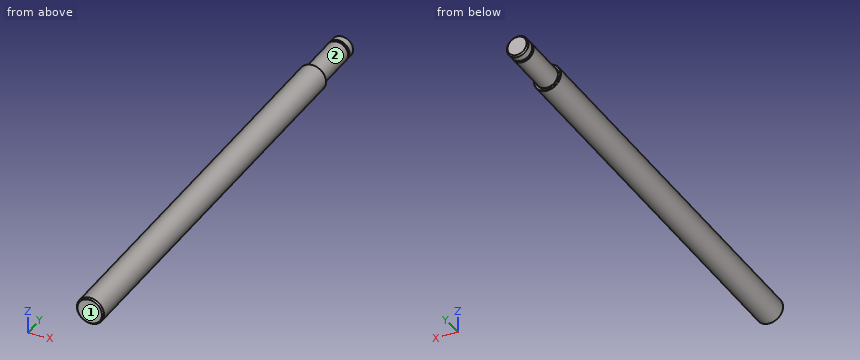
from build123d import *

# Parameters (mm, degrees)
RESSALTO_EXTRUS_O1_DEPTH      = 94
RESSALTO_EXTRUS_O1_DEPTH_BACK = 82
ESBO_O1_R                     = 5
ESBO_O2_R                     = 14
ESBO_O2_R_2                   = 4
CORTE_EXTRUS_O1_DEPTH         = 21
CHANFRO1_SIZE                 = 0.5
FILETE1_R                     = 0.25
CHANFRO2_SIZE                 = 0.5
CORTE_EXTRUS_O2_START         = -3
ESBO_O3_R                     = 13.5
ESBO_O3_R_2                   = 3.5
CORTE_EXTRUS_O2_DEPTH         = 1


with BuildPart() as part:
    # Esboço1 → Ressalto-extrusão1 (new, two sides: drawn at the far end of the back side and taken through both)
    with BuildSketch(Plane(origin=(0, 0, 0), x_dir=(1, 0, 0), z_dir=(0, 1, 0)).offset(-RESSALTO_EXTRUS_O1_DEPTH_BACK)):
        with Locations(Location((0, 0, 0), (0, 0, 270))):
            Circle(ESBO_O1_R)
    extrude(amount=RESSALTO_EXTRUS_O1_DEPTH + RESSALTO_EXTRUS_O1_DEPTH_BACK)

    # Esboço2 → Corte-extrusão1 (cut)
    with BuildSketch(Plane(origin=(0, 94, 0), x_dir=(1, 0, 0), z_dir=(0, 1, 0))):
        Circle(ESBO_O2_R)
        with Locations(Location((0, 0, 0), (0, 0, 270))):
            Circle(ESBO_O2_R_2, mode=Mode.SUBTRACT)
    extrude(amount=-CORTE_EXTRUS_O1_DEPTH, mode=Mode.SUBTRACT)

    # Chanfro1
    chanfro1_edges = [part.edges().sort_by_distance(p)[0] for p in [
        (0, 94, -4),
    ]]
    chamfer(chanfro1_edges, length=CHANFRO1_SIZE)

    # Filete1
    filete1_edges = [part.edges().sort_by_distance(p)[0] for p in [
        (0, 73, -5),
        (0, 73, -4),
    ]]
    fillet(filete1_edges, radius=FILETE1_R)

    # Chanfro2
    chanfro2_edges = [part.edges().sort_by_distance(p)[0] for p in [
        (0, -82, -5),
    ]]
    chamfer(chanfro2_edges, length=CHANFRO2_SIZE)

    # Esboço3 → Corte-extrusão2 (cut)
    with BuildSketch(Plane(origin=(0, 94, 0), x_dir=(1, 0, 0), z_dir=(0, 1, 0)).offset(CORTE_EXTRUS_O2_START)):
        Circle(ESBO_O3_R)
        with Locations(Location((0, 0, 0), (0, 0, 270))):
            Circle(ESBO_O3_R_2, mode=Mode.SUBTRACT)
    extrude(amount=-CORTE_EXTRUS_O2_DEPTH, mode=Mode.SUBTRACT)


solid = part.part
For this review, take the finished solid that the model builds, in its own axes (mm). Face numbers are marked on the shaded views. A direction names the side the tool comes from. Coordinates: 2 decimals unless noted, no trailing zeros. Loops run counter-clockwise (first coordinate to the right, second up) from the corner with the lowest first, then second, coordinate; pieces in that order, holes last. Notation, with made-up numbers: (-18, 53) - (10, 53) arc R28 cw to (10, 83) - close; hole circle Ø8 at (9.25, -10). An arc over 180 degrees is marked (long way). Return JSON: item names as keys, results as strings.
Item 1: Take a section at A-A (z = 0). Give the boundary of the cut face in (x, y).
Determined:
{"outline": "(-5, -81.5) - (-4.5, -82) - (4.5, -82) - (5, -81.5) - (5, 72.75) arc R0.25 ccw to (4.75, 73) - (4.25, 73) arc R0.25 cw to (4, 73.25) - (4, 90) - (3.5, 90) - (3.5, 91) - (4, 91) - (4, 93.5) - (3.5, 94) - (-3.5, 94) - (-4, 93.5) - (-4, 91) - (-3.5, 91) - (-3.5, 90) - (-4, 90) - (-4, 73.25) arc R0.25 cw to (-4.25, 73) - (-4.75, 73) arc R0.25 ccw to (-5, 72.75) - close"}
Item 2: Take a section at B-B (x = 0). Give the boundary of the cut face in (y, z), then the cut area to 3 significant figures.
Determined:
{"outline": "(-82, -4.5) - (-81.5, -5) - (72.75, -5) arc R0.25 ccw to (73, -4.75) - (73, -4.25) arc R0.25 cw to (73.25, -4) - (90, -4) - (90, -3.5) - (91, -3.5) - (91, -4) - (93.5, -4) - (94, -3.5) - (94, 3.5) - (93.5, 4) - (91, 4) - (91, 3.5) - (90, 3.5) - (90, 4) - (73.25, 4) arc R0.25 cw to (73, 4.25) - (73, 4.75) arc R0.25 ccw to (72.75, 5) - (-81.5, 5) - (-82, 4.5) - close", "area": "1,720 mm2"}
Item 3: Take a section at D-D (y = 75.5). Give the boundary of the cut face in (x, z), then the cut area to 3 significant figures.
Determined:
{"outline": "circle Ø8 at (0, 0)", "area": "50.3 mm2"}
Item 4: Insertion check: pin 1 (1.5 mm diameter, centred on x = 4, y = -30, fed in from +Z); pin 2 (5 mm diameter, centred on y = 10.5, z = 2, fed in from +X); pin 3 (2 mm diameter, centred on x = 3.5, y = -10.5, fed in from +Z); pin 4 (5 mm diameter, centred on y = -3, z = -3, fed in from -X). Each pin has a flat end and moves straight along its axis. Give the tip position at first contact, or say it passes through.
Determined:
{"pin 1": "stops at z = 3.8", "pin 2": "stops at x = 5", "pin 3": "stops at z = 4.33", "pin 4": "stops at x = -4.97"}
Item 5: For line 1 (Y direction, x = -3, z = 3); line 2 (Y direction, x = 2.75, z = -2.5); line 3 (Y direction, x = -3.25, z = -1.5), list the stretches that pass through material, from the lowest coordinate up.
Determined:
{"line 1": "y = -82 to 73", "line 2": "y = -82 to 90, 91 to 93.78", "line 3": "y = -82 to 90, 91 to 93.92"}
Item 6: For the marked faces 1 and 2, list the 3-axis set-ups (+Z, -Z, +X, -X, +Y, -Y) from which the entire face can be reached by the end or side of a thin tool; tool diameter is ignored.
Determined:
{"face 1": "+Z, -Z, +X, -X, -Y", "face 2": "+Y"}
Item 7: Take a section at C-C (y = -1.5). Give the boundary of the cut face in (x, z).
Determined:
{"outline": "circle Ø10 at (0, 0)"}
